```python
from build123d import *

# Parameters (mm, degrees)
SKETCH1_R           = 4.7625
BOSS_EXTRUDE1_DEPTH = 73.66
SKETCH2_R           = 3.81
BOSS_EXTRUDE2_DEPTH = 1.016
SKETCH3_R           = 4.7625
BOSS_EXTRUDE3_DEPTH = 25.654
SKETCH4_R           = 3.81
BOSS_EXTRUDE4_DEPTH = 1.016
SKETCH5_R           = 4.7625
BOSS_EXTRUDE5_DEPTH = 25.654


with BuildPart() as part:
    # Sketch1 → Boss-Extrude1 (new body)
    with BuildSketch(Plane.XY):
        Circle(SKETCH1_R)
    extrude(amount=BOSS_EXTRUDE1_DEPTH)

    # Sketch2 → Boss-Extrude2 (add)
    with BuildSketch(Plane(origin=(0, 0, 0), x_dir=(-1, 0, 0), z_dir=(0, 0, -1))):
        Circle(SKETCH2_R)
    extrude(amount=BOSS_EXTRUDE2_DEPTH)

    # Sketch3 → Boss-Extrude3 (add)
    with BuildSketch(Plane(origin=(0, 0, -1.016), x_dir=(-1, 0, 0), z_dir=(0, 0, -1))):
        Circle(SKETCH3_R)
    extrude(amount=BOSS_EXTRUDE3_DEPTH)

    # Sketch4 → Boss-Extrude4 (add)
    with BuildSketch(Plane.XY.offset(73.66)):
        Circle(SKETCH4_R)
    extrude(amount=BOSS_EXTRUDE4_DEPTH)

    # Sketch5 → Boss-Extrude5 (add)
    with BuildSketch(Plane.XY.offset(74.676)):
        Circle(SKETCH5_R)
    extrude(amount=BOSS_EXTRUDE5_DEPTH)


solid = part.part
```
Can you work these out from the model? Positions are in its coordinate system, mm. A direction names the side the tool comes from. Coordinates: 2 decimals unless noted, no trailing zeros. Write each loop counter-clockwise with the first axis right and the second up, starting at its lowest first coordinate (ties: lowest second). Pieces come first, ordered by that corner, then holes. Notation, with made-up numbers: M -3.5,-30 L 53.5,-30 A19 cw 53.5,0 Z; hole C -21,74 d8. An arc over 180 degrees is marked long. Answer as CSV lines item,"result".
Item 1: Imagine slicing it at A-A on x = -2.5. List the corners of the cut face in (y, z) for me, plus the area to 3 significant figures.
Geometry results:
outline,"M -4.05,-26.67 L 4.05,-26.67 L 4.05,-1.02 L 2.88,-1.02 L 2.88,0 L 4.05,0 L 4.05,73.66 L 2.88,73.66 L 2.88,74.68 L 4.05,74.68 L 4.05,100.33 L -4.05,100.33 L -4.05,74.68 L -2.88,74.68 L -2.88,73.66 L -4.05,73.66 L -4.05,0 L -2.88,0 L -2.88,-1.02 L -4.05,-1.02 Z"
area,"1,020 mm2"
Item 2: Please list where these lines run through material, in increasing order: line 1 along Z through (x, y) = (-3.5, -2.5); line 2 along Y through (x, z) = (-0.5, 70); line 3 along Y through (x, z) = (-0.25, 64.5).
Geometry results:
line 1,"z = -26.67 to -1.02, 0 to 73.66, 74.68 to 100.33"
line 2,"y = -4.74 to 4.74"
line 3,"y = -4.76 to 4.76"
Item 3: We'd pull the mould along Z, two halves only. Please class faces 3 (the flat face through (1, 4, 73.66)), 4 (the cylindrical face through (-3.78, -2.9, 87.32)), 5 (the flat face through (0, 0, -26.67)): +Z half, -Z half, draft (parallel to the pull), parting line (faces both ways), or undercut.
Geometry results:
face 3,"undercut"
face 4,"draft"
face 5,"-Z half"
Item 4: I'm going to push a flat-ended pin straight in: P1, Ø1, axis at y = -1, z = 83, coming from the +X side. Where does the tip first touch, or does it pass through?
Geometry results:
P1,"stops at x = 4.74"
Item 5: On a 3-axis mill with a long thin cutter (end or side, diameter ignored), from which of +Z, -Z, +X, -X, +Y, -Y can I reach the whole of each face in a straight line? I mean faces 1 (the cylindrical face through (-0.83, -3.72, 74.16)), 2 (the cylindrical face through (3.78, -2.9, -13.66)). Say none if no direction works.
Geometry results:
face 1,"none"
face 2,"+Z, -Z"
Item 6: Imagine slicing it at C-C on x = 2.75. List the corners of the cut face in (y, z) for me, plus the area to 3 significant figures.
Geometry results:
outline,"M -3.89,-26.67 L 3.89,-26.67 L 3.89,-1.02 L 2.64,-1.02 L 2.64,0 L 3.89,0 L 3.89,73.66 L 2.64,73.66 L 2.64,74.68 L 3.89,74.68 L 3.89,100.33 L -3.89,100.33 L -3.89,74.68 L -2.64,74.68 L -2.64,73.66 L -3.89,73.66 L -3.89,0 L -2.64,0 L -2.64,-1.02 L -3.89,-1.02 Z"
area,"983 mm2"
Item 7: Imagine slicing it at B-B on z = 53.5. List the corners of the cut face in (x, y) for me (1 decimal).
Geometry results:
outline,"C 0,0 d9.5"
